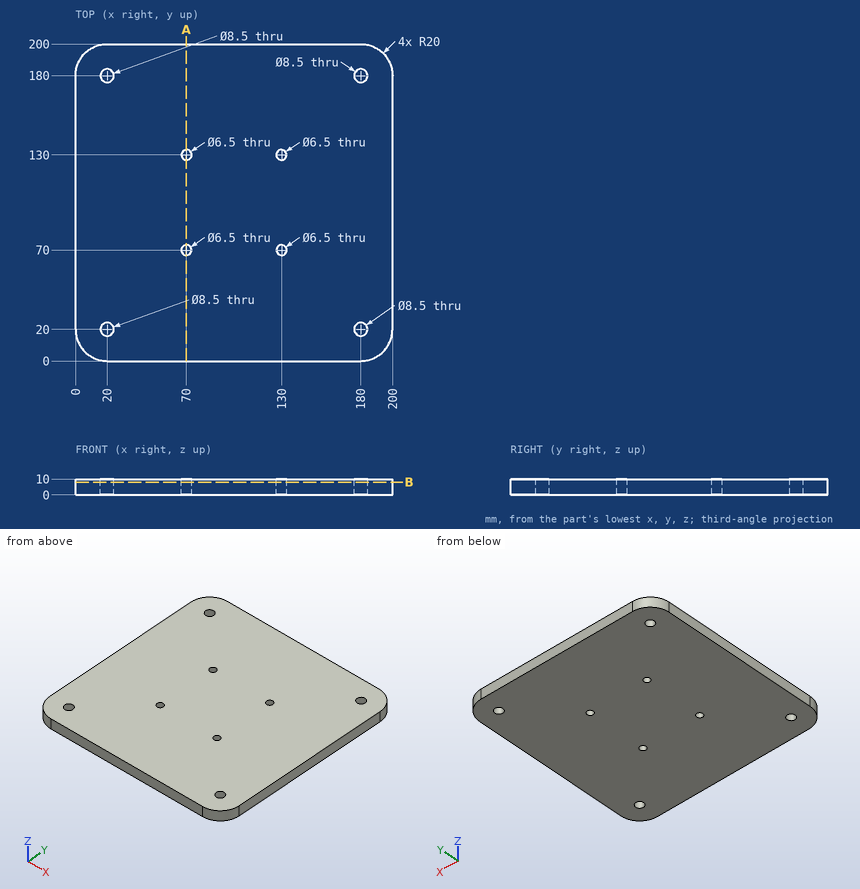
Source: three-view drawing plus pictorial views. Frame: mm from the lowest corner of the part. Round coordinates to 2 decimals unless told otherwise and drop trailing zeros. Write each loop counter-clockwise with the first axis right and the second up, starting at its lowest first coordinate (ties: lowest second). Pieces come first, ordered by that corner, then holes. Notation, with made-up numbers: M 81.25,-3.5 L 132.25,-3.5 A28 cw 132.25,34.5 Z; hole C -0.75,44 d8. An arc over 180 degrees is marked long. Use CSV: the item, a comma, the result in double quotes. Start each with the question number.
Q1. First-contact query: P1, Ø7, axis at x = 180, y = 20, coming from the +Z side. Flat tip, straight axial feed; report the tip coordinate or a pass-through.
Q2. Cut plane A-A on x = 70. Output: boundary loops of the cut face in (y, z).
Q3. Line query: line 1 (X direction, y = 180, z = 9.25); line 2 (Y direction, x = 70, z = 6). Output: solid intervals per line, ascending. Write a range as from..to.
Q4. Cut plane B-B on z = 8. Count the separate pieces of the cut face and the enclosed holes in it, plus the area to 3 significant figures.
Results found:
1,P1,"through"
2,outline,"M 0,0 L 66.75,0 L 66.75,10 L 0,10 Z; M 73.25,0 L 126.75,0 L 126.75,10 L 73.25,10 Z; M 133.25,0 L 200,0 L 200,10 L 133.25,10 Z"
3,line 1,"0..15.75, 24.25..175.75, 184.25..200"
3,line 2,"0..66.75, 73.25..126.75, 133.25..200"
4,separate pieces,"1"
4,enclosed holes,"8"
4,area,"39,300 mm^2"
